The listing builds one solid part. Answer for the finished solid, in the listing's coordinates (mm). A direction names the side the tool comes from. Coordinates: 2 decimals unless noted, no trailing zeros. Order: outer loops, then holes, each group sorted by start corner. A loop starts at its lowest first (then second) coordinate and runs counter-clockwise, first axis right, second up. Notation, with made-up numbers: (-11, 2.25) -> (32, 2.25) arc R32 cw to (32, 30.25) -> close; hole circle Ø9 at (3.5, 6.5). An arc over 180 degrees is marked (long way). Write each question's results on one line, items separated by ' | '. Start each with the question number.
(1) Determine the mould class of faces 4 (the face through (-1.5, 0.07, 0.99)), 5 (the face through (-2.5, -3.12, 0.99)), 6 (the face through (4, -4, 1)) for opening direction X: +X half, -X half, draft (parallel to the pull), parting line (faces both ways), or undercut.
(2) The part is cut by section A-A, the plane y = 0. Give the vertices of the cut face in (x, z), then the cut area to 3 significant figures.
(3) The part is cut by section B-B, the plane z = 0.95. Give the vertices of the cut face in (x, y).
(4) Given pin 1 (1 mm diameter, centred on y = 2.5, z = 2, fed in from +X); pin 2 (0.8 mm diameter, centred on x = -3, z = 1, fed in from +Y); pin 3 (0.6 mm diameter, centred on y = 2.5, z = 1, fed in from -X), each flat-ended and moving along its own axis, determine where each tip first touches the part or whether it passes through.
(5) A tool of negligible diameter and unlimited length cuts with its end or side. For faces 1 (the face through (2.995, 1, 1)), 2 (the face through (-6, -0.8, 1)), 3 (the face through (-3, 3.2, 1)), from which of +Z, -Z, +X, -X, +Y, -Y can it reach the whole face along a straight path? Write none if from no direction.
(6) The part is cut by section C-C, the plane x = 0.25. Give the vertices of the cut face in (y, z).
(7) Straight lines are drawn through the part: L1, parallel to Y at x = 0, z = 0.8; L2, parallel to Y at x = 4.5, z = 1.4; L3, parallel to Y at x = -4.5, z = 0.4. For each, find the intervals that lie inside material, in ascending order.
(8) The part is cut by section D-D, the plane x = -5.75. Give the vertices of the cut face in (y, z).
```python
from build123d import *

# Parameters (mm, degrees)
SKETCH1_R           = 1.5
BOSS_EXTRUDE1_DEPTH = 2


with BuildPart() as part:
    # Sketch1 → Boss-Extrude1 (new body)
    with BuildSketch(Plane.XY):
        with BuildLine():
            Line((7.72, -4), (0, -4))
            ThreePointArc((0, -4), (-2.529822128, -3.098386677), (-3.919183588, -0.8))
            Line((-3.919183588, -0.8), (-8.919183588, -0.8))
            Line((-8.919183588, -0.8), (-8.919183588, 1.2))
            Line((-8.919183588, 1.2), (-3.919183588, 1.2))
            Line((-3.919183588, 1.2), (-3.919183588, 3.2))
            Line((-3.919183588, 3.2), (-2.4, 3.2))
            ThreePointArc((-2.4, 3.2), (0.404610957, 3.979483631), (2.994944065, 2.651473185))
            Line((2.994944065, 2.651473185), (2.994944065, -1.348526815))
            Line((2.994944065, -1.348526815), (7.72, -1.348526815))
            Line((7.72, -1.348526815), (7.72, -4))
        make_face()
        Circle(SKETCH1_R, mode=Mode.SUBTRACT)
    extrude(amount=BOSS_EXTRUDE1_DEPTH)


solid = part.part
```
Established:
1) face 4: undercut | face 5: -X half | face 6: draft
2) outline: (-8.92, 0) -> (-1.5, 0) -> (-1.5, 2) -> (-8.92, 2) -> close; (1.5, 0) -> (2.99, 0) -> (2.99, 2) -> (1.5, 2) -> close | area: 17.8 mm^2
3) outline: (-8.92, -0.8) -> (-3.92, -0.8) arc R4 ccw to (0, -4) -> (7.72, -4) -> (7.72, -1.35) -> (2.99, -1.35) -> (2.99, 2.65) arc R4 ccw to (-2.4, 3.2) -> (-3.92, 3.2) -> (-3.92, 1.2) -> (-8.92, 1.2) -> close; hole circle Ø3 at (0, 0)
4) pin 1: stops at x = 2.99 | pin 2: stops at y = 3.2 | pin 3: stops at x = -3.92
5) face 1: +Z, -Z, +X, +Y | face 2: +Z, -Z, -X, -Y | face 3: +Z, -Z, -X, +Y
6) outline: (-4, 0) -> (-1.48, 0) -> (-1.48, 2) -> (-4, 2) -> close; (1.48, 0) -> (3.99, 0) -> (3.99, 2) -> (1.48, 2) -> close
7) L1: y = -4 to -1.5, 1.5 to 4 | L2: y = -4 to -1.35 | L3: y = -0.8 to 1.2
8) outline: (-0.8, 0) -> (1.2, 0) -> (1.2, 2) -> (-0.8, 2) -> close
